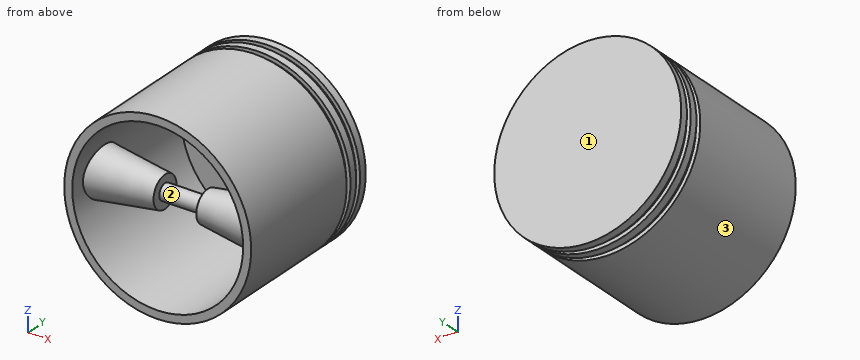
from build123d import *

# Parameters (mm, degrees)
SKETCH_1_R           = 35
EXTRUDE_1_DEPTH      = 60
SHELL_1_T            = -3
SKETCH_2_R           = 3
EXTRUDE_2_DEPTH      = 8
EXTRUDE_3_REACH      = 83.695
EXTRUDE_3_END_RADIUS = 32
SKETCH_3_R           = 6
EXTRUDE_3_DRAFT      = -8
SKETCH_4_W           = 1.5
SKETCH_4_H           = 2


with BuildPart() as part:
    # Sketch 1 → Extrude 1 (new body)
    with BuildSketch(Plane(origin=(0, 0, 0), x_dir=(1, 0, 0), z_dir=(0, 1, 0))):
        with Locations(Location((0, 0, 0), (0, 0, 270))):
            Circle(SKETCH_1_R)
    extrude(amount=EXTRUDE_1_DEPTH)

    # Shell 1
    shell_1_openings = [part.faces().sort_by_distance(p)[0] for p in [
        (0, 0, 0),
    ]]
    offset(amount=SHELL_1_T, openings=shell_1_openings, kind=Kind.INTERSECTION)



with BuildPart() as body_2:
    # Sketch 2 → Extrude 2 (new body)
    with BuildSketch(Plane(origin=(0, 0, 0), x_dir=(0, 0, -1), z_dir=(1, 0, 0))):
        with Locations((0, 15)):
            Circle(SKETCH_2_R)
    extrude_2 = extrude(amount=-EXTRUDE_2_DEPTH)


with BuildPart() as part_1:
    add(part.part)

    add(body_2.part)  # Extrude 3 merges body 2
    # Extrude 3: up to this cylinder (the profile starts inside it)
    extrude_3_end = Plane(origin=(0, 15, 0), z_dir=(0, -1, 0)) * Cylinder(EXTRUDE_3_END_RADIUS, 232.39, mode=Mode.PRIVATE)



with BuildPart() as extrude_3_long_prism_1:
    # Sketch 3 → Extrude 3 (the long prism of profile 1, to be tilted and cut off)
    with BuildSketch(Plane.ZY.offset(8)):
        with Locations((0, 15)):
            Circle(SKETCH_3_R)
    extrude(amount=EXTRUDE_3_REACH)
    extrude_3_tool1_sides = [extrude_3_long_prism_1.faces().sort_by_distance(p)[0] for p in [
        (-49.8475, 15, -6),
    ]]
    draft(extrude_3_tool1_sides, Plane.ZY.offset(8), EXTRUDE_3_DRAFT)  # the draft: side faces tilted about the start plane


with BuildPart() as part_2:
    add(part_1.part)
    extrude_3_tool1 = extrude_3_long_prism_1.part & extrude_3_end
    extrude_3 = extrude_3_tool1.solids().sort_by_distance((-8, 15, 0))[0]
    add(extrude_3)

    # Mirror 1: Extrude 2, Extrude 3 across plane
    add(extrude_2.mirror(Plane(origin=(0, 15, 0), x_dir=(0, 0, 1), z_dir=(1, 0, 0))))
    add(extrude_3.mirror(Plane(origin=(0, 15, 0), x_dir=(0, 0, 1), z_dir=(1, 0, 0))))

    # Sketch 4 → Cut-Revolve 1 (revolve, cut)
    with BuildSketch(Plane.XY, mode=Mode.PRIVATE) as cut_revolve_1_sk:
        with Locations((-34.25, 56)):
            Rectangle(SKETCH_4_W, SKETCH_4_H)
        with Locations((-34.25, 51)):
            Rectangle(SKETCH_4_W, SKETCH_4_H)
    revolve(cut_revolve_1_sk.sketch.rotate(Axis((0, 47.542228421, 0), (0, 1, 0)), 270), axis=Axis((0, 47.542228421, 0), (0, 1, 0)), mode=Mode.SUBTRACT)


solid = part_2.part
Build history of the part. All positions in model axes, mm. Face numbers are marked on the shaded views. Coordinates: 2 decimals unless noted, no trailing zeros. Order: outer loops, then holes, each group sorted by start corner. A loop starts at its lowest first (then second) coordinate and runs counter-clockwise, first axis right, second up. Notation, with made-up numbers: (25.25, 54.5) - (78.25, 54.5) arc R22 ccw to (78.25, 63.5) - close; hole circle Ø4 at (-23, 56.5). An arc over 180 degrees is marked (long way). Put each result on its own line as item: value.
1. Saw through at B-B (y = 44.5). Write the cut outline in (x, z).
Answer sheet:
outline: circle Ø70 at (0, 0); hole circle Ø64 at (0, 0)
2. Saw through at A-A (x = 0). Write the cut outline in (y, z).
Answer sheet:
outline: (0, -35) - (50, -35) - (50, -33.5) - (52, -33.5) - (52, -35) - (55, -35) - (55, -33.5) - (57, -33.5) - (57, -35) - (60, -35) - (60, 35) - (57, 35) - (57, 33.5) - (55, 33.5) - (55, 35) - (52, 35) - (52, 33.5) - (50, 33.5) - (50, 35) - (0, 35) - (0, 32) - (57, 32) - (57, -32) - (0, -32) - close; circle Ø6 at (15, 0)
3. Saw through at D-D (x = 13.5). Write the cut outline in (y, z).
Answer sheet:
outline: (0, -32.29) - (50, -32.29) - (50, -30.66) - (52, -30.66) - (52, -32.29) - (55, -32.29) - (55, -30.66) - (57, -30.66) - (57, -32.29) - (60, -32.29) - (60, 32.29) - (57, 32.29) - (57, 30.66) - (55, 30.66) - (55, 32.29) - (52, 32.29) - (52, 30.66) - (50, 30.66) - (50, 32.29) - (0, 32.29) - (0, 29.01) - (57, 29.01) - (57, -29.01) - (0, -29.01) - close; circle Ø13.55 at (15, 0)
4. Pull direction Y, two halves, no side cores. Call the marked faces 1, 2 and 3: pulls with the +Y half, pulls with the -Y half, needs draft (parallel to the pull), parting line crosses it, or undercut.
Answer sheet:
face 1: pulls with the +Y half
face 2: undercut
face 3: needs draft
5. Drop flat-ended pins along their axis: P1, Ø8, axis at x = 15.5, y = 12.5, coming from the +Z side; P2, Ø10, axis at y = 22.5, z = 23.5, coming from the -X side; P3, Ø6, axis at y = 17, z = 1, coming from the -X side. Give the stop position or say it passes through.
Answer sheet:
P1: stops at z = 33.06
P2: stops at x = -29.71
P3: stops at x = -35
6. Saw through at C-C (z = -14.5). Write the cut outline in (x, y).
Answer sheet:
outline: (-31.86, 0) - (-28.53, 0) - (-28.53, 57) - (28.53, 57) - (28.53, 0) - (31.86, 0) - (31.86, 50) - (30.2, 50) - (30.2, 52) - (31.86, 52) - (31.86, 55) - (30.2, 55) - (30.2, 57) - (31.86, 57) - (31.86, 60) - (-31.86, 60) - (-31.86, 57) - (-30.2, 57) - (-30.2, 55) - (-31.86, 55) - (-31.86, 52) - (-30.2, 52) - (-30.2, 50) - (-31.86, 50) - close
7. Probe line 1 along X through (y, z) = (29.5, 0); line 2 along Z through (x, y) = (-5.5, 13.5). List the from-to ranges inside material, lowest first. Write a range as [from, to].
Answer sheet:
line 1: x = [-35, -32], [32, 35]
line 2: z = [-34.57, -31.52], [-2.6, 2.6], [31.52, 34.57]
